Autodesk Inventor part; units mm, degrees
ref_plane "YZ Plane" through (0, 0, 0) normal (1, 0, 0) x (0, 1, 0)
ref_plane "XZ Plane" through (0, 0, 0) normal (0, 1, 0) x (-1, 0, 0)
ref_plane "XY Plane" through (0, 0, 0) normal (0, 0, 1) x (1, 0, 0)
sketch "草圖1" plane through (0, 0, 0) normal (0, 1, 0) x (-1, 0, 0)
  line L0 (0, 0) -> (-35, 0)
  line L1 (-35, 0) -> (-35, -40)
  line L2 (-35, -40) -> (0, -40)
  line L3 (0, -40) -> (0, 0)
  line L4 (0, -40) -> (0, -39)
  line L5 (0, -39) -> (-35, -39)
  line L6 (-35, -39) -> (-35, -40)
  line L7 (-35, -40) -> (0, -40)
  line L8 (0, 0) -> (0, -1)
  line L9 (0, -1) -> (-35, -1)
  line L10 (-35, -1) -> (-35, 0)
  line L11 (-35, 0) -> (0, 0)
  dimension "d0" = 35
  dimension "d1" = 40
  dimension "d19" = 1
  dimension "d20" = 1
extrude "擠出1" add sketch "草圖1" along normal blind 10 contours L3 L5 L1 L9
sketch "草圖2" plane through (0, 10, 0) normal (0, 1, 0) x (1, 0, 0)
  line L0 (0, 0) -> (0, 20)
  line L1 (0, 20) -> (17.5, 20)
  line L2 (17.5, 20) -> (17.5, 0)
  line L3 (17.5, 0) -> (0, 0)
  line L4 (17.5, 20) -> (2.5, 20)
  line L5 (2.5, 20) -> (3.2342, 24.6353)
  line L6 (3.2342, 24.6353) -> (5.3647, 28.8168)
  line L7 (5.3647, 28.8168) -> (8.6832, 32.1353)
  line L8 (8.6832, 32.1353) -> (12.8647, 34.2658)
  line L9 (12.8647, 34.2658) -> (17.5, 35)
  line L10 (17.5, 35) -> (22.1353, 34.2658)
  line L11 (22.1353, 34.2658) -> (26.3168, 32.1353)
  line L12 (26.3168, 32.1353) -> (29.6353, 28.8168)
  line L13 (29.6353, 28.8168) -> (31.7658, 24.6353)
  line L14 (31.7658, 24.6353) -> (32.5, 20)
  line L15 (32.5, 20) -> (31.7658, 15.3647)
  line L16 (31.7658, 15.3647) -> (29.6353, 11.1832)
  line L17 (29.6353, 11.1832) -> (26.3168, 7.8647)
  line L18 (26.3168, 7.8647) -> (22.1353, 5.7342)
  line L19 (22.1353, 5.7342) -> (17.5, 5)
  line L20 (17.5, 5) -> (12.8647, 5.7342)
  line L21 (12.8647, 5.7342) -> (8.6832, 7.8647)
  line L22 (8.6832, 7.8647) -> (5.3647, 11.1832)
  line L23 (5.3647, 11.1832) -> (3.2342, 15.3647)
  line L24 (3.2342, 15.3647) -> (2.5, 20)
  dimension "d7" = 17.5
  dimension "d8" = 20
  dimension "d9" = 15
extrude "擠出2" add sketch "草圖2" along normal blind 0.5 contours L5 L6 L7 L8 L9 L10 L11 L12 L13 L14 L15 L16 L17 L18 L19 L2 L1 | L1 L2 L20 L21 L22 L23 L24
sketch "草圖3" plane through (35, 0, 0) normal (1, 0, 0) x (0, 0, -1)
  line L0 (40, 0) -> (40, 10)
  line L1 (1, 10) -> (39, 10)
  line L2 (40, 0) -> (40, 10)
  line L3 (40, 10) -> (0, 10)
  line L4 (0, 10) -> (0, 0)
  line L5 (0, 0) -> (40, 0)
  line L6 (1, 0) -> (1, 10)
  line L7 (0, 10) -> (1, 10)
  line L8 (1, 10) -> (1, 0)
  line L9 (1, 0) -> (0, 0)
  line L10 (0, 0) -> (0, 10)
  line L11 (39, 0) -> (39, 10)
  line L12 (39, 10) -> (40, 10)
  line L13 (40, 10) -> (40, 0)
  line L14 (40, 0) -> (39, 0)
  line L15 (39, 0) -> (39, 10)
  point P0 (0, 0)
extrude "擠出3" add sketch "草圖3" along normal blind 1.5 contours L5 L6 L1 L11
sketch "草圖4" plane through (0, 0, -40) normal (-1, 0, 0) x (0, 0, 1)
  line L0 (0, 10) -> (40, 10)
  line L1 (40, 10) -> (40, 0)
  line L2 (40, 0) -> (0, 0)
  line L3 (0, 0) -> (0, 10)
  line L4 (1, 0) -> (1, 10)
  line L5 (1, 0) -> (1, 10)
  line L6 (39, 0) -> (39, 10)
  line L7 (1, 10) -> (39, 10)
  line L8 (39, 10) -> (39, 0)
  line L9 (0, 10) -> (1, 10)
  line L10 (1, 10) -> (1, 0)
  line L11 (1, 0) -> (0, 0)
  line L12 (0, 0) -> (0, 10)
  line L13 (39, 10) -> (40, 10)
  line L14 (40, 10) -> (40, 0)
  line L15 (40, 0) -> (39, 0)
  line L16 (39, 0) -> (39, 10)
extrude "擠出4" add sketch "草圖4" along normal blind 1.5 contours L0 L6 L2 L4
chamfer "倒角3" distance 2 angle 45 4 edges at (36.5, 5, -1) (36.5, 5, -39) (-1.5, 5, -39) (-1.5, 5, -1)
properties part number "樓上跟尖下"
Input: part model. Units: mm. Frame: model coordinates. A direction names the side the tool comes from. Give positions to 0.01 mm unless a question says otherwise; leave off trailing zeros. Loops run counter-clockwise (first coordinate to the right, second up) from the corner with the lowest first, then second, coordinate; pieces in that order, holes last. Notation, with made-up numbers: M 38,-30 L 70,-30 A29 cw 70,-1 Z; hole C 33,41 d7. An arc over 180 degrees is marked long. Use CSV: the item, a comma, the result in double quotes.
(1) Section B-B, the plane x = 27. Return loops of the section in (y, z).
Outcome:
outline,"M 0,-39 L 10,-39 L 10,-31.45 L 10.5,-31.45 L 10.5,-8.55 L 10,-8.55 L 10,-1 L 0,-1 Z"
(2) Pin query (flat end, axial travel): P1, Ø3, axis at x = 15, z = -32.5, coming from the -Y side; P2, Ø1.5, axis at x = 6, z = -8.5, coming from the +Y side. Return the tip coordinate at first contact, or that it passes through.
Outcome:
P1,"stops at y = 0"
P2,"stops at y = 10"
(3) Set-up query: faces 1 (the face through (7, 10.25, -30.45)), 2 (the face through (28, 10.25, -9.55)), 3 (the face through (4.314, 10.246, -13.245)). Return all of +Z, -Z, +X, -X, +Y, -Y with unobstructed straight access to the full face (end or side cutting, diameter ignored); none if empty.
Outcome:
face 1,"-Z, -X, +Y"
face 2,"+Z, +X, +Y"
face 3,"+Z, -X, +Y"
(4) Material intervals for L1, parallel to Y at x = 6, z = -34; L2, parallel to Z at x = 0, y = 9.5, sorted ascending. Write a range as [from, to].
Outcome:
L1,"y = [0, 10]"
L2,"z = [-38.5, -1.5]"
(5) Section A-A, the plane z = -33.5. Return loops of the section in (x, y), plus the area to 3 significant figures.
Outcome:
outline,"M -1.5,0 L 36.5,0 L 36.5,10 L 23.64,10 L 23.64,10.5 L 11.36,10.5 L 11.36,10 L -1.5,10 Z"
area,"386 mm²"
